Here's how the part is built. I have some questions about the finished solid (model axes, mm). Coordinates: 2 decimals unless noted, no trailing zeros. Write each loop counter-clockwise with the first axis right and the second up, starting at its lowest first coordinate (ties: lowest second). Pieces come first, ordered by that corner, then holes.
Item 1: If we mould it in two halves opening along Y, with no side actions, what happens to faces 1 (the face through (-0.767, -2.435, -1)), 2 (the face through (3.14, 5.52, -1)), 3 (the face through (3.21, -5.48, -1)), 4 (the face through (6.35, 0, -1))? For each: pulls with the +Y half, pulls with the -Y half, needs draft (parallel to the pull), parting line crosses it, or undercut.
Item 2: Please list where these lines run through material, in increasing order: line 1 (Y direction, x = 0, z = -13.5); line 2 (X direction, y = 0, z = -17.5); line 3 (Y direction, x = 0.25, z = 2).
Item 3: I want a section at B-B (z = 44.5). Please give me the cut outline in (x, y).
Item 4: I want a section at A-A (y = 0). Please give me the cut outline in (x, z).
Item 5: I'm going to push flat-ended pins straight in: P1, Ø1, axis at x = -1.5, z = -47, coming from the +Y side; P2, Ø1.5, axis at y = -5, z = 42, coming from the +X side. Where does each tip first touch, or does it pass through?
Autodesk Inventor part; units mm, degrees
ref_plane "YZ Plane" through (0, 0, 0) normal (1, 0, 0) x (0, 1, 0)
ref_plane "XZ Plane" through (0, 0, 0) normal (0, 1, 0) x (-1, 0, 0)
ref_plane "XY Plane" through (0, 0, 0) normal (0, 0, 1) x (1, 0, 0)
sketch "Sketch1" plane through (0, 0, 0) normal (0, 0, 1) x (1, 0, 0)
  line L0 (-6.35, -3.6662) -> (-6.35, 3.6662)
  line L1 (-6.35, 3.6662) -> (0, 7.3323)
  line L2 (0, 7.3323) -> (6.35, 3.6662)
  line L3 (6.35, 3.6662) -> (6.35, -3.6662)
  line L4 (6.35, -3.6662) -> (0, -7.3323)
  line L5 (0, -7.3323) -> (-6.35, -3.6662)
  point P0 (0, 0)
  point P1 (0, 0)
  dimension "Size" = 12.7
extrude "Extrusion1" add sketch "Sketch1" along normal mid plane 142.875
sketch "Sketch3" plane through (0, 0, 71.4375) normal (0, 0, 1) x (1, 0, 0)
  line L0 (-6.35, 3.6662) -> (0, 7.3323) construction
  line L1 (0, 7.3323) -> (6.35, 3.6662) construction
  line L2 (6.35, 3.6662) -> (6.35, -3.6662) construction
  line L3 (6.35, -3.6662) -> (0, -7.3323) construction
  line L4 (0, -7.3323) -> (-6.35, -3.6662) construction
  line L5 (-6.35, -3.6662) -> (-6.35, 3.6662) construction
  point P0 (0, 0)
hole "Hole1" at (0, 0, 71.4375) direction (0, 0, -1) diameter 5.1054 end through all
sketch "Sketch4" plane through (0, 0, 71.4375) normal (0, 0, 1) x (1, 0, 0)
  circle A0 centre (0, 0) radius 2.5527 construction
  line L0 (-6.35, 3.6662) -> (0, 7.3323) construction
  line L1 (0, 7.3323) -> (6.35, 3.6662) construction
  line L2 (6.35, 3.6662) -> (6.35, -3.6662) construction
  line L3 (6.35, -3.6662) -> (0, -7.3323) construction
  line L4 (0, -7.3323) -> (-6.35, -3.6662) construction
  line L5 (-6.35, -3.6662) -> (-6.35, 3.6662) construction
  circle A1 centre (0, 0) radius 6.8771
  circle A2 centre (0, 0) radius 8.89
  dimension "thunder" = 13.7541
  dimension "d16" = 17.78
extrude "Extrusion3" cut sketch "Sketch4" against normal through all
equation "\"bearing\" = 25.4"
properties part number "GP4-010" material "Aluminum 6061"
Answer:
1. face 1: undercut
1. face 2: pulls with the +Y half
1. face 3: pulls with the -Y half
1. face 4: needs draft
2. line 1: y = -6.88 to -2.55, 2.55 to 6.88
2. line 2: x = -6.35 to -2.55, 2.55 to 6.35
2. line 3: y = -6.87 to -2.54, 2.54 to 6.87
3. outline: (-6.35, -2.64) arc R6.88 ccw to (-5.46, -4.18) - (-0.89, -6.82) arc R6.88 ccw to (0.89, -6.82) - (5.46, -4.18) arc R6.88 ccw to (6.35, -2.64) - (6.35, 2.64) arc R6.88 ccw to (5.46, 4.18) - (0.89, 6.82) arc R6.88 ccw to (-0.89, 6.82) - (-5.46, 4.18) arc R6.88 ccw to (-6.35, 2.64) - close; hole circle Ø5.11 at (0, 0)
4. outline: (-6.35, -71.44) - (-2.55, -71.44) - (-2.55, 71.44) - (-6.35, 71.44) - close; (2.55, -71.44) - (6.35, -71.44) - (6.35, 71.44) - (2.55, 71.44) - close
5. P1: stops at y = 6.75
5. P2: stops at x = 5.34
